Design review of the part built by this model. Coordinates are the model's own, in mm. Face numbers are marked on the shaded views. A direction names the side the tool comes from. Give positions to 0.01 mm unless a question says otherwise; leave off trailing zeros. Write each loop counter-clockwise with the first axis right and the second up, starting at its lowest first coordinate (ties: lowest second). Pieces come first, ordered by that corner, then holes. Notation, with made-up numbers: M 67.5,81.25 L 80.5,81.25 A19 ccw 80.5,113.25 Z; hole C 12,44.5 d10. An arc over 180 degrees is marked long. Use a Markdown table: item, result. Add a question column.
```python
from build123d import *

# Parameters (mm, degrees)
F1_DEPTH = 25.4


with BuildPart() as f1:
    # F0 (on Front) → F1 (new body)
    with BuildSketch(Plane.XZ):
        Polygon((-71.842049, 71.842049), (0, 0), (71.842049, 71.842049), (53.881537, 89.802561), (-53.881537, 89.802561), align=None)
        with BuildLine():
            Line((17.325188, 23.675188), (0, 6.35))
            Line((0, 6.35), (-17.325188, 23.675188))
            ThreePointArc((-17.325188, 23.675188), (0, 18.840947), (17.325188, 23.675188))
        make_face(mode=Mode.SUBTRACT)
        with BuildLine():
            Line((-27.88843, 37.371293), (-43.441594, 53.192612))
            Line((-43.441594, 53.192612), (-33.519749, 49.70656))
            Line((-33.519749, 49.70656), (26.547641, 43.538928))
            ThreePointArc((26.547641, 43.538928), (27.826581, 36.254042), (20.916322, 33.617079))
            Line((20.916322, 33.617079), (-10.190004, 37.103135))
            ThreePointArc((-10.190004, 37.103135), (-18.94585, 43.399421), (-27.88843, 37.371293))
        make_face(mode=Mode.SUBTRACT)
        with BuildLine():
            ThreePointArc((-46.700488, 83.452561), (-53.089277, 75.177991), (-56.225224, 65.20548))
            Line((-56.225224, 65.20548), (-62.861793, 71.842049))
            Line((-62.861793, 71.842049), (-51.251281, 83.452561))
            Line((-51.251281, 83.452561), (-46.700488, 83.452561))
        make_face(mode=Mode.SUBTRACT)
        with BuildLine():
            Line((53.881537, 67.93008), (53.881537, 83.452561))
            Line((53.881537, 83.452561), (65.492049, 71.842049))
            Line((65.492049, 71.842049), (49.96895, 56.31895))
            ThreePointArc((49.96895, 56.31895), (42.256735, 58.261775), (34.860542, 55.33788))
            Line((34.860542, 55.33788), (-24.575694, 60.914379))
            ThreePointArc((-24.575694, 60.914379), (-38.321211, 59.825174), (-40.998805, 73.351301))
            ThreePointArc((-40.998805, 73.351301), (-3.816385, 83.83065), (31.390447, 67.93008))
            Line((31.390447, 67.93008), (53.881537, 67.93008))
        make_face(mode=Mode.SUBTRACT)
        Polygon((37.845217, 80.521145), (35.590284, 83.452561), (39.761905, 83.452561), align=None, mode=Mode.SUBTRACT)
    extrude(amount=-F1_DEPTH)


solid = f1.part
```
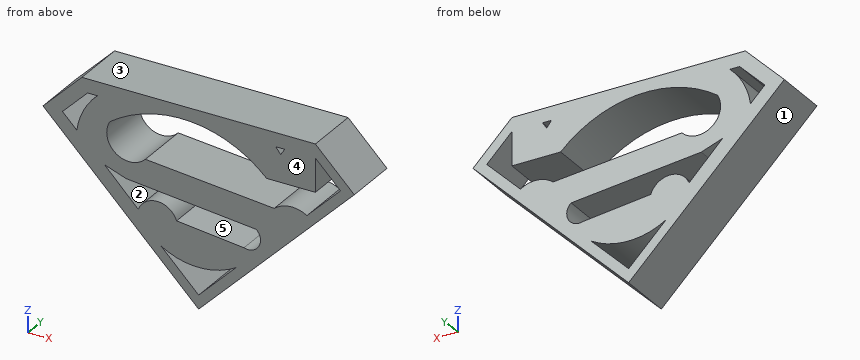
(1) Machinability: for the marked faces 4 and 5, which of the approach directions +Z, -Z, +X, -X, +Y, -Y give a long, thin tool a straight path to every point of the face, cutting with its end or side? Answer none if there is none.
(2) The part is to be moulded in two halves that separate along Z. For the marked faces 1, 2 and 3, say which applies: released by +Z, released by -Z, zero draft, split by the parting line, or undercut.
(3) Add section B-B on y = 15.25. Give the number of separate pieces and of enclosed holes in the cut face, then the cut area to 3 significant figures.
(4) Wall thickness on L1, parallel to Z at x = -2, y = 15; L2, parallel to Z at x = -18, y = 11; L3, parallel to X at y = 6.5, z = 75.5: over which ranges is each line inside the solid? List them lowest first.
(5) For pin 1 (6 mm diameter, centred on y = 23, z = 41, fed in from -X); pin 2 (12 mm diameter, centred on x = -17.5, z = 77, fed in from -Y); pin 3 (1.4 mm diameter, centred on x = -48, y = 13.5, fed in from -Z); pin 4 (5 mm diameter, centred on y = 21, z = 80, fed in from -X), all flat-tipped, find the tip position at first contact; note any pin that passes through.
(6) Add section C-C on x = -7. Give the boundary of the cut face in (y, z), then the cut area to 3 significant figures.
(7) Add section D-D on x = -31.5. Give the boundary of the cut face in (y, z).
(8) Add section A-A on z = 14. Give the boundary of the cut face in (x, y).
From the geometry:
| question | item | result |
|---|---|---|
| 1 | face 4 | +Z, -Z, +X, -X, -Y |
| 1 | face 5 | +Y, -Y |
| 2 | face 1 | released by -Z |
| 2 | face 2 | undercut |
| 2 | face 3 | released by +Z |
| 3 | separate pieces | 1 |
| 3 | enclosed holes | 5 |
| 3 | area | 4,620 mm^2 |
| 4 | L1 | z = 2 to 8.35, 18.9 to 36.19, 46.47 to 58.8, 83.67 to 89.8 |
| 4 | L2 | z = 18 to 43.34, 48.11 to 60.3, 83.1 to 89.8 |
| 4 | L3 | x = -68.18 to -59.2, -52.92 to -37.79, 21.73 to 53.88, 61.83 to 68.18 |
| 5 | pin 1 | stops at x = -44 |
| 5 | pin 2 | passes through |
| 5 | pin 3 | stops at z = 47.3 |
| 5 | pin 4 | stops at x = -66.18 |
| 6 | outline | M 0,7 L 25.4,7 L 25.4,13.35 L 0,13.35 Z; M 0,19.58 L 25.4,19.58 L 25.4,36.75 L 0,36.75 Z; M 0,46.98 L 25.4,46.98 L 25.4,59.27 L 0,59.27 Z; M 0,83.98 L 25.4,83.98 L 25.4,89.8 L 0,89.8 Z |
| 6 | area | 1,060 mm^2 |
| 7 | outline | M 0,31.5 L 25.4,31.5 L 25.4,41.05 L 0,41.05 Z; M 0,49.5 L 25.4,49.5 L 25.4,57.74 L 0,57.74 Z; M 0,78.87 L 25.4,78.87 L 25.4,89.8 L 0,89.8 Z |
| 8 | outline | M -14,0 L -7.65,0 L -7.65,25.4 L -14,25.4 Z; M 7.65,0 L 14,0 L 14,25.4 L 7.65,25.4 Z |
